Could you check a few things on this model? Use its own coordinates, in mm. Face numbers are marked on the shaded views. Round coordinates to 2 decimals unless told otherwise and drop trailing zeros. Write each loop counter-clockwise with the first axis right and the second up, starting at its lowest first coordinate (ties: lowest second). Pieces come first, ordered by that corner, then holes. Notation, with made-up numbers: (74, -35.75) -> (95, -35.75) arc R12 cw to (95, -16.75) -> close; hole circle Ø11 at (10, -1). An arc over 180 degrees is marked (long way). Answer as CSV lines item,"result". Start each with the question number.
Q1. If we mould it in two halves opening along Y, with no side actions, what happens to the marked faces 1, 2 and 3? For each: pulls with the +Y half, pulls with the -Y half, needs draft (parallel to the pull), parting line crosses it, or undercut.
Q2. Will these pins go through, and if not, where does the flat tip stop? pin 1 Ø1 at (x, y) = (-19, -15) entering from -Z; pin 2 Ø1.5 at (x, z) = (-9.5, 1) entering from +Y; pin 3 Ø1.5 at (y, z) = (7.5, 2) entering from +X; pin 4 Ø5 at (x, y) = (-10.5, 10) entering from +Z.
Q3. Imagine slicing it at C-C on z = 0.8. Please give me the cut outline in (x, y), and give its area (3 significant figures).
Q4. Imagine slicing it at D-D on y = -16. Please give me the cut outline in (x, z), and give its area (3 significant figures).
Q5. Imagine slicing it at A-A on x = -13. Please give me the cut outline in (y, z).
Q6. If I drill on line 1 (X direction, y = 10, z = 1.9); line 2 (Y direction, x = -10.5, z = 2); line 3 (Y direction, x = -8.75, z = 2.45), over which ranges is the centre line in solid material (lowest first)? Write a range as [from, to].
Q7. Imagine slicing it at B-B on y = 8. Please give me the cut outline in (x, z).
from build123d import *

# Parameters (mm, degrees)
F1_DEPTH = 3


with BuildPart() as f1:
    # F0 (on Top) → F1 (new body)
    with BuildSketch(Plane.XY):
        with BuildLine():
            ThreePointArc((-6.5559468113, 9.3333333333), (-5.6054684353, 8.9564392374), (-4.6905249807, 8.5))
            ThreePointArc((-4.6905249807, 8.5), (-4.5478218224, 9.2439742451), (-4.5, 10))
            ThreePointArc((-4.5, 10), (-11.2560257549, 15.9521781776), (-16.3094750193, 8.5))
            ThreePointArc((-16.3094750193, 8.5), (-15.3945315647, 8.9564392374), (-14.4440531887, 9.3333333333))
            ThreePointArc((-14.4440531887, 9.3333333333), (-10.8345050411, 13.9859887578), (-6.5, 10))
            ThreePointArc((-6.5, 10), (-6.5140112422, 9.6654949589), (-6.5559468113, 9.3333333333))
        make_face()
        with BuildLine():
            ThreePointArc((-16.3094750193, 8.5), (-10.5, 4), (-4.6905249807, 8.5))
            ThreePointArc((-4.6905249807, 8.5), (-5.6054684353, 8.9564392374), (-6.5559468113, 9.3333333333))
            ThreePointArc((-6.5559468113, 9.3333333333), (-10.5, 6), (-14.4440531887, 9.3333333333))
            ThreePointArc((-14.4440531887, 9.3333333333), (-15.3945315647, 8.9564392374), (-16.3094750193, 8.5))
        make_face()
        with BuildLine():
            ThreePointArc((-1.3321595662, 0), (-0.8273722771, 1.9611409085), (0, 3.8094750193))
            ThreePointArc((0, 3.8094750193), (-2.0147186258, 6.4852813742), (-4.6905249807, 8.5))
            ThreePointArc((-4.6905249807, 8.5), (-10.5, 4), (-16.3094750193, 8.5))
            ThreePointArc((-16.3094750193, 8.5), (-20.8371587061, 4.094518019), (-22.5, -2))
            ThreePointArc((-22.5, -2), (-22.3914639986, -3.2113902714), (-22.253495394, -4.4197822265))
            ThreePointArc((-22.253495394, -4.4197822265), (-12.3070188109, -13.8631649663), (0, -7.8094750193))
            ThreePointArc((0, -7.8094750193), (-1.3291298387, -4.0178422283), (-1.3321595662, 0))
        make_face()
        with BuildLine():
            ThreePointArc((0, -7.8094750193), (0.6272994629, -6.4925723882), (1.0901824777, -5.1092877211))
            Line((1.0901824777, -5.1092877211), (-1.3321595662, 0))
            ThreePointArc((-1.3321595662, 0), (-1.3291298387, -4.0178422283), (0, -7.8094750193))
        make_face()
        with BuildLine():
            Line((1.7156613405, -6.4285693978), (1.0901824777, -5.1092877211))
            ThreePointArc((1.0901824777, -5.1092877211), (0.6272994629, -6.4925723882), (0, -7.8094750193))
            ThreePointArc((0, -7.8094750193), (0.3883389068, -8.4617574959), (0.8171440868, -9.0881803987))
            Line((0.8171440868, -9.0881803987), (1.7156613405, -6.4285693978))
        make_face()
        with BuildLine():
            ThreePointArc((0.8171440868, -9.0881803987), (0.3883389068, -8.4617574959), (0, -7.8094750193))
            ThreePointArc((0, -7.8094750193), (-12.3070188109, -13.8631649663), (-22.253495394, -4.4197822265))
            ThreePointArc((-22.253495394, -4.4197822265), (-15.0403231441, -24.6576201784), (0, -40))
            Line((0, -40), (2.3193413737, -30.6764196892))
            Line((2.3193413737, -30.6764196892), (-3.3150132865, -21.3193659027))
            Line((-3.3150132865, -21.3193659027), (0.8171440868, -9.0881803987))
        make_face()
        with BuildLine():
            Line((-1.3321595662, 0), (0, 3.8094750193))
            ThreePointArc((0, 3.8094750193), (-0.8273722771, 1.9611409085), (-1.3321595662, 0))
        make_face()
    extrude(amount=F1_DEPTH)


solid = f1.part
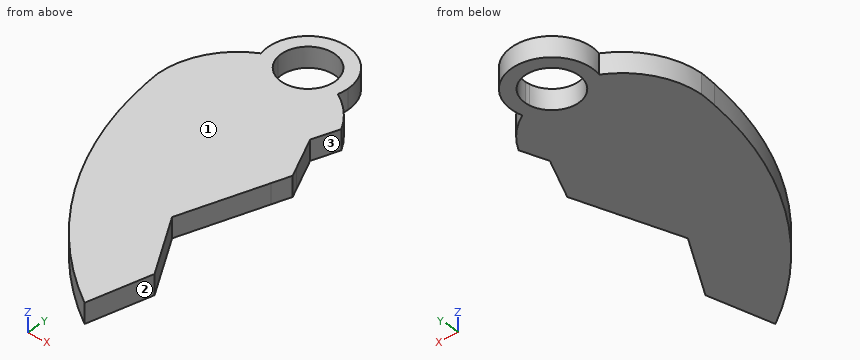
Checks:
1,face 1,"needs draft"
1,face 2,"pulls with the -Y half"
1,face 3,"undercut"
2,pin 1,"z = 0"
2,pin 2,"y = 15.99"
2,pin 3,"x = -2.29"
2,pin 4,"through"
3,outline,"(-22.5, -2) arc R50 ccw to (0, -40) -> (2.32, -30.68) -> (-3.32, -21.32) -> (1.72, -6.43) -> (-1.33, 0) -> (0, 3.81) arc R12 ccw to (-4.69, 8.5) arc R6 ccw (long way) to (-16.31, 8.5) arc R12 ccw to start; hole circle Ø8 at (-10.5, 10)"
3,area,"806 mm^2"
4,outline,"(-19.35, 0) -> (-1.52, 0) -> (-1.52, 3) -> (-19.35, 3) -> close"
4,area,"53.5 mm^2"
5,outline,"(-27.67, 0) -> (6.88, 0) -> (6.88, 3) -> (-27.67, 3) -> close; (13.12, 0) -> (15.45, 0) -> (15.45, 3) -> (13.12, 3) -> close"
6,line 1,"[-16.5, -14.5], [-6.5, -4.5]"
6,line 2,"[-30.81, 6], [14, 16]"
6,line 3,"[-32.74, 6.4], [13.6, 15.74]"
7,outline,"(-17.13, 0) -> (-13.96, 0) -> (-13.96, 3) -> (-17.13, 3) -> close; (-7.04, 0) -> (-3.87, 0) -> (-3.87, 3) -> (-7.04, 3) -> close"
